```python
from build123d import *

# Parameters (mm, degrees)
F0_R     = 5
F1_DEPTH = 2.5
F3_DEPTH = 10


# Not quite as in the source:
# - a feature names something its author has since deleted; it is built from what else it names


with BuildPart() as f1:
    # F0 (on Top) → F1 (new body, symmetric)
    with BuildSketch(Plane.XY):
        with BuildLine():
            ThreePointArc((2.8545027599, -6.0492269011), (0, -6.146341392), (-2.8545027599, -6.0492269011))
            ThreePointArc((-2.8545027599, -6.0492269011), (-30.6911152935, 7.182149369), (-42, 35.853658608))
            ThreePointArc((-42, 35.853658608), (-50.5591908622, 43.8340912767), (-57.9218263949, 34.7380123518))
            Line((-57.9218263949, 34.7380123518), (-48.2619276413, -33.853658608))
            Line((-48.2619276413, -33.853658608), (-42, -33.853658608))
            Line((-42, -33.853658608), (-42, -29.853658608))
            Line((-42, -29.853658608), (-28, -29.853658608))
            Line((-28, -29.853658608), (-28, -33.853658608))
            Line((-28, -33.853658608), (28, -33.853658608))
            Line((28, -33.853658608), (28, -29.853658608))
            Line((28, -29.853658608), (42, -29.853658608))
            Line((42, -29.853658608), (42, -33.853658608))
            Line((42, -33.853658608), (48.2619276413, -33.853658608))
            Line((48.2619276413, -33.853658608), (57.9218263949, 34.7380123518))
            ThreePointArc((57.9218263949, 34.7380123518), (50.5591908622, 43.8340912767), (42, 35.853658608))
            ThreePointArc((42, 35.853658608), (30.6911152935, 7.182149369), (2.8545027599, -6.0492269011))
        make_face()
        with Locations((-50, 35.853658608)):
            Circle(F0_R, mode=Mode.SUBTRACT)
        with Locations((50, 35.853658608)):
            Circle(F0_R, mode=Mode.SUBTRACT)
    extrude(amount=F1_DEPTH, both=True)

    # F2 (on face) → F3 (join, symmetric)
    with BuildSketch(Plane.XY.offset(2.5)):
        with BuildLine():
            Line((48.2619276413, -33.853658608), (50.2816638994, -33.853658608))
            Line((50.2816638994, -33.853658608), (59.9022829936, 34.4591007877))
            ThreePointArc((59.9022829936, 34.4591007877), (50.6989885778, 45.8291994439), (40, 35.853658608))
            ThreePointArc((40, 35.853658608), (0, -4.146341392), (-40, 35.853658608))
            ThreePointArc((-40, 35.853658608), (-50.6989885778, 45.8291994439), (-59.9022829936, 34.4591007877))
            Line((-59.9022829936, 34.4591007877), (-50.2816638994, -33.853658608))
            Line((-50.2816638994, -33.853658608), (-48.2619276413, -33.853658608))
            Line((-48.2619276413, -33.853658608), (-57.9218263949, 34.7380123518))
            ThreePointArc((-57.9218263949, 34.7380123518), (-50.5591908622, 43.8340912767), (-42, 35.853658608))
            ThreePointArc((-42, 35.853658608), (0, -6.146341392), (42, 35.853658608))
            ThreePointArc((42, 35.853658608), (50.5591908622, 43.8340912767), (57.9218263949, 34.7380123518))
            Line((57.9218263949, 34.7380123518), (48.2619276413, -33.853658608))
        make_face()
    extrude(amount=F3_DEPTH, both=True)


solid = f1.part
```
Source: CAD feature listing. Evaluate the final solid. Frame: model axes, mm. A direction names the side the tool comes from. Give positions to 0.01 mm unless a question says otherwise; leave off trailing zeros. Loops run counter-clockwise (first coordinate to the right, second up) from the corner with the lowest first, then second, coordinate; pieces in that order, holes last. Notation, with made-up numbers: (51, 60.5) -> (104, 60.5) arc R31 cw to (104, 96.5) -> close; hole circle Ø1 at (84, 64). An arc over 180 degrees is marked (long way). Use a Markdown table: item, result. Add a question column.
(1) Access query for faces 1 (the face through (28, -32, 0)), 2 (the face through (-1, -12, -2.5)), 3 (the face through (-1, -12, 2.5)). Directions: +Z, -Z, +X, -X, +Y, -Y. A direction counts if a zero-diameter tool reaches every point of the face in a straight line with its end or side. Return the directions, or none.
(2) Ray query, line 1 (Y direction, x = -50, z = -1.5); line 2 (X direction, y = 3, z = 7); line 3 (X direction, y = 4, z = -3.75). Return the intervals inside material, ascending.
(3) Section query B-B (y = 17). Output: boundary loops of the cut face in (x, z), then the cut area to 3 significant figures.
(4) Section query A-A (x = 0). Output: boundary loops of the cut face in (y, z), then the cut area to 3 significant figures.
(5) Section query D-D (y = -15). Output: boundary loops of the cut face in (x, z), then the cut area to 3 significant figures.
(6) Section query C-C (z = 9.5). Output: boundary loops of the cut face in (x, y).
(7) First-contact query: pin 1 Ø2.5 at (x, z) = (37, 1) entering from -Y; pin 2 Ø1.5 at (y, z) = (29, 0) entering from +X; pin 3 Ø3 at (x, z) = (-47.5, 9.5) entering from -Y; pin 4 Ø2 at (y, z) = (-32, 0) entering from -X. Flat tips, straight axial feed; report the tip coordinate or a pass-through.
Checked values:
| question | item | result |
|---|---|---|
| 1 | face 1 | +Z, -Z, -Y |
| 1 | face 2 | -Z |
| 1 | face 3 | +Z |
| 2 | line 1 | -33.85 to 30.85, 40.85 to 45.85 |
| 2 | line 2 | -55.47 to -53.45, -26.17 to -22.82, 22.82 to 26.17, 53.45 to 55.47 |
| 2 | line 3 | -55.61 to -53.59, -27.37 to -24.19, 24.19 to 27.37, 53.59 to 55.61 |
| 3 | outline | (-57.44, -7.5) -> (-55.42, -7.5) -> (-55.42, -2.5) -> (-37.53, -2.5) -> (-37.53, -7.5) -> (-35.28, -7.5) -> (-35.28, 12.5) -> (-37.53, 12.5) -> (-37.53, 2.5) -> (-55.42, 2.5) -> (-55.42, 12.5) -> (-57.44, 12.5) -> close; (35.28, -7.5) -> (37.53, -7.5) -> (37.53, -2.5) -> (55.42, -2.5) -> (55.42, -7.5) -> (57.44, -7.5) -> (57.44, 12.5) -> (55.42, 12.5) -> (55.42, 2.5) -> (37.53, 2.5) -> (37.53, 12.5) -> (35.28, 12.5) -> close |
| 3 | area | 350 mm^2 |
| 4 | outline | (-33.85, -2.5) -> (-6.15, -2.5) -> (-6.15, -7.5) -> (-4.15, -7.5) -> (-4.15, 12.5) -> (-6.15, 12.5) -> (-6.15, 2.5) -> (-33.85, 2.5) -> close |
| 4 | area | 179 mm^2 |
| 5 | outline | (-52.94, -7.5) -> (-50.92, -7.5) -> (-50.92, -2.5) -> (50.92, -2.5) -> (50.92, -7.5) -> (52.94, -7.5) -> (52.94, 12.5) -> (50.92, 12.5) -> (50.92, 2.5) -> (-50.92, 2.5) -> (-50.92, 12.5) -> (-52.94, 12.5) -> close |
| 5 | area | 590 mm^2 |
| 6 | outline | (-59.9, 34.46) -> (-50.28, -33.85) -> (-48.26, -33.85) -> (-57.92, 34.74) arc R8 cw (long way) to (-42, 35.85) arc R42 ccw to (42, 35.85) arc R8 cw (long way) to (57.92, 34.74) -> (48.26, -33.85) -> (50.28, -33.85) -> (59.9, 34.46) arc R10 ccw (long way) to (40, 35.85) arc R40 cw to (-40, 35.85) arc R10 ccw (long way) to start |
| 7 | pin 1 | y = -29.85 |
| 7 | pin 2 | x = 59.24 |
| 7 | pin 3 | y = -33.85 |
| 7 | pin 4 | x = -50.68 |
